Autodesk Inventor part; units mm, degrees
ref_plane "Work Plane1" through (0, -14.2875, 0) normal (0, 1, 0) x (-1, 0, 0)
ref_plane "YZ Plane" through (0, 0, 0) normal (1, 0, 0) x (0, 1, 0)
ref_plane "XY Plane" through (0, 0, 0) normal (0, 0, 1) x (1, 0, 0)
sketch "Sketch1" plane through (0, 0, 0) normal (0, 0, 1) x (1, 0, 0)
  circle A0 centre (0, 0) radius 14.2875
  circle A1 centre (0, 0) radius 12.065
  dimension "d0" = 28.575
  dimension "d1" = 24.13
extrude "Extrusion1" add sketch "Sketch1" along normal blind 13.97
sketch "Sketch2" plane through (0, 0, 13.97) normal (0, 0, 1) x (1, 0, 0)
  circle A0 centre (0, 0) radius 14.2875
  circle A1 centre (0, 0) radius 14.2875
extrude "Extrusion2" add sketch "Sketch2" along normal blind 2.54
sketch "Sketch3" plane through (0, 0, 16.51) normal (0, 0, 1) x (1, 0, 0)
  circle A0 centre (0, 0) radius 14.2875
  circle A1 centre (0, 0) radius 7.9375
  dimension "d6" = 15.875
extrude "Extrusion3" add sketch "Sketch3" along normal blind 12.7 contours A1
thread "Thread1"
ref_plane "Work Plane1" through (0, -14.2875, 0) normal (0, 1, 0) x (-1, 0, 0)
sketch "Sketch4" plane through (0, -14.2875, 0) normal (0, 1, 0) x (-1, 0, 0)
  line L0 (-14.2875, 16.51) -> (14.2875, 16.51)
  line L1 (-14.2875, 0) -> (14.2875, 0)
  circle A0 centre (0, 8.255) radius 5.3975
  point P0 (0, 0)
  dimension "d12" = 10.795
  dimension "d13" = 8.255
extrude "Extrusion4" cut sketch "Sketch4" along normal blind 12.7
sketch "Sketch5" plane through (0, 0, 29.21) normal (0, 0, 1) x (1, 0, 0)
  circle A0 centre (0, 0) radius 7.9375
  circle A1 centre (0, 0) radius 4.1275
  dimension "d16" = 8.255
extrude "Extrusion5" cut sketch "Sketch5" against normal through all contours A1
properties part number "1in Actuator Top Cap 1764"
Read the model definition and answer for the solid it produces. Units are mm, in the model's axes. A direction names the side the tool comes from. Coordinates: 2 decimals unless noted, no trailing zeros. Loops run counter-clockwise (first coordinate to the right, second up) from the corner with the lowest first, then second, coordinate; pieces in that order, holes last. Notation, with made-up numbers: (6.25, -14) -> (20.25, -14) arc R24 ccw to (20.25, 23) -> close; hole circle Ø4 at (39.25, 17.25). An arc over 180 degrees is marked (long way). Write item = value, one per line. Start each with the question number.
1) The part is cut by section B-B, the plane y = 0. Determine the outline of the cut face in (x, z) (1 decimal).
2) The part is cut by section A-A, the plane x = 0. State how many separate pieces and enclosed holes the cut face has, plus the area to 3 significant figures.
3) Find the intervals of material crossed by L1, parallel to Y at x = -0.25, z = 27.25; L2, parallel to Z at x = 0, y = -12.4; L3, parallel to Y at x = -2.5, z = 13.75, in increasing order. Write a range as from..to.
4) The part is cut by section C-C, the plane z = 17.5. Determine the outline of the cut face in (x, y) (1 decimal).
5) For faces 1 (the face through (-3.097, 13.948, 8.139)), 2 (the face through (0, -5, 13.97)), 3 (the face through (6, -6, 16.51)), determine the directions among +Z, -Z, +X, -X, +Y, -Y from which every point of the face is accessible in a straight line to the end or side of a thin tool.
6) The mould has two halves that part along X. Classify faces 4 (the face through (5.567, 10.704, 6.887)), 5 (the face through (-1.72, 7.75, 22.77)), 6 (the face through (-2.902, -12.563, 3.704)), 7 (the face through (-12, -3, 0)): pulls with the +X half, pulls with the -X half, needs draft (parallel to the pull), parting line crosses it, or undercut.
7) Given P1, Ø2, axis at y = 7.5, z = 7.5, coming from the -X side; P2, Ø5, axis at y = -5, z = 16, coming from the -X side; P3, Ø4, axis at x = 6, y = 7, coming from the -Z side, each flat-ended and moving along its own axis, determine where each tip first touches the part or whether it passes through.
8) The part is cut by section D-D, the plane y = -7.5. Determine the outline of the cut face in (x, z).
Result:
q1.outline = (-14.3, 0) -> (-12.1, 0) -> (-12.1, 14) -> (-4.1, 14) -> (-4.1, 29.2) -> (-7.9, 29.2) -> (-7.9, 16.5) -> (-14.3, 16.5) -> close; (4.1, 14) -> (12.1, 14) -> (12.1, 0) -> (14.3, 0) -> (14.3, 16.5) -> (7.9, 16.5) -> (7.9, 29.2) -> (4.1, 29.2) -> close
q2.separate_pieces = 3
q2.enclosed_holes = 0
q2.area = 186 mm²
q3.L1 = -7.93..-4.12, 4.12..7.93
q3.L2 = 0..2.86, 13.65..16.51
q3.L3 = -14.07..-11.8, 11.8..14.07
q4.outline = circle Ø15.9 at (0, 0); hole circle Ø8.3 at (0, 0)
q5.face_1 = +Z, -Z
q5.face_2 = -Z
q5.face_3 = +Z
q6.face_4 = undercut
q6.face_5 = parting line crosses it
q6.face_6 = undercut
q6.face_7 = needs draft
q7.P1 = -12.72
q7.P2 = -14.07
q7.P3 = 13.97
q8.outline = (-12.16, 0) -> (-9.45, 0) -> (-9.45, 13.97) -> (9.45, 13.97) -> (9.45, 0) -> (12.16, 0) -> (12.16, 16.51) -> (2.6, 16.51) -> (2.6, 29.21) -> (-2.6, 29.21) -> (-2.6, 16.51) -> (-12.16, 16.51) -> close
